For this review, take the finished solid that the model builds, in its own axes (mm). A direction names the side the tool comes from. Round coordinates to 2 decimals unless told otherwise and drop trailing zeros. Write each loop counter-clockwise with the first axis right and the second up, starting at its lowest first coordinate (ties: lowest second). Pieces come first, ordered by that corner, then holes. Notation, with made-up numbers: (15, -8.75) - (33, -8.75) arc R26 cw to (33, 11.25) - close; hole circle Ø2 at (9.25, 33.5). An arc over 180 degrees is marked (long way). One line per item, written item: value. Start each with the question number.
Q1. Tool access review of faces 1 (the face through (-24, -40, -7)), 2 (the face through (71.5, -0.6, -81.1)): name each direction out of +Z, -Z, +X, -X, +Y, -Y from which nothing blocks a thin tool from reaching the whole face with its end or side.
Q2. Add section A-A on x = 8. Write out the cut boundary in (y, z).
Q3. Add section D-D on z = -49. Write out the cut boundary in (x, y).
Q4. Add section C-C on x = -41.5. Write out the cut boundary in (y, z).
Q5. Add section B-B on y = -21. Write out the cut boundary in (x, z).
Q6. For probe 1 along Y at (x, z) = (-41.5, -0.7); probe 2 along Y at (x, z) = (9.5, -155), list the stretches that pass through material, from the lowest coordinate up.
Q7. Mouldability with a two-part tool opening along Y and no side actions: class faces 3 (the face through (-64.1, -10.9, -0.5)), 4 (the face through (62, -41, -7)), 5 (the face through (-1, -21, 0)) as +Y half, -Y half, draft (parallel to the pull), parting line (faces both ways), or undercut.
Q8. Clearance check with flat-ended pins moving along their axes: pin 1 Ø0.8 at (x, z) = (8.5, -0.5) entering from +Y (3 decimals); pin 2 Ø10 at (x, z) = (64, -4) entering from -Y; pin 3 Ø1.1 at (x, y) = (-24, -40.5) entering from -Z. State where each tip first meets the part, or that it passes through.
```python
from build123d import *

# Parameters (mm, degrees)
BASE_FLANGE1_START       = -71.5
BASE_FLANGE1_DEPTH       = 143
SKETCH6_W                = 39
SKETCH6_H                = 165
CUT_EXTRUDE1_DEPTH       = 1
SKETCH7_W                = 4
SKETCH7_H                = 46
CUT_EXTRUDE2_DEPTH       = 10
SKETCH8_R                = 2.6
CUT_EXTRUDE3_DEPTH       = 1
SKETCH9_W                = 16
SKETCH9_H                = 2
SKETCH9_W_2              = 8
SKETCH9_H_2              = 4.5
CUT_EXTRUDE4_DEPTH       = 185.66523766
SKETCH10_R               = 1.25
CUT_EXTRUDE5_DEPTH       = 1
EDGE_FLANGE1_START       = 56
EDGE_FLANGE1_DEPTH       = 13
EDGE_FLANGE1_2_DEPTH     = 0.5
EDGE_FLANGE1_START_2     = 68.5
EDGE_FLANGE1_3_DEPTH     = 0.5
EDGE_FLANGE1_START_3     = 56.5
EDGE_FLANGE1_4_OUTLINE_W = 1
EDGE_FLANGE1_4_OUTLINE_H = 9
EDGE_FLANGE1_4_DEPTH     = 12
EDGE_FLANGE2_START       = -30
EDGE_FLANGE2_DEPTH       = 13
EDGE_FLANGE2_2_DEPTH     = 0.5
EDGE_FLANGE2_START_2     = -17.5
EDGE_FLANGE2_3_DEPTH     = 0.5
EDGE_FLANGE2_START_3     = -29.5
EDGE_FLANGE2_4_OUTLINE_W = 1
EDGE_FLANGE2_4_OUTLINE_H = 9
EDGE_FLANGE2_4_DEPTH     = 12
SKETCH17_R               = 1.25
CUT_EXTRUDE6_DEPTH       = 1
FILLET1_R                = 2


# Read off the part's stored shape, not the designer's step: Base-Flange1, Edge-Flange1, Edge-Flange2
with BuildPart() as part:
    # Base-Flange1 outline → Base-Flange1 (new body)
    with BuildSketch(Plane(origin=(0, 0, 0), x_dir=(0, 0, -1), z_dir=(1, 0, 0)).offset(BASE_FLANGE1_START)):
        with BuildLine():
            Line((1, -1), (165, -1))
            Line((165, -1), (165, 0))
            Line((165, 0), (1, 0))
            ThreePointArc((1, 0), (0.292893219, -0.292893219), (0, -1))
            Line((0, -1), (0, -42))
            Line((0, -42), (1, -42))
            Line((1, -42), (1, -1))
        make_face()
    extrude(amount=BASE_FLANGE1_DEPTH)

    # Sketch6 → Cut-Extrude1 (cut)
    with BuildSketch(Plane(origin=(0, 0, 0), x_dir=(1, 0, 0), z_dir=(0, 1, 0))):
        with Locations((-52, 82.5)):
            Rectangle(SKETCH6_W, SKETCH6_H)
    extrude(amount=-CUT_EXTRUDE1_DEPTH, mode=Mode.SUBTRACT)

    # Sketch7 → Cut-Extrude2 (cut)
    with BuildSketch(Plane(origin=(0, 0, 0), x_dir=(1, 0, 0), z_dir=(0, 1, 0))):
        with Locations((-30.5, 142)):
            Rectangle(SKETCH7_W, SKETCH7_H)
    extrude(amount=-CUT_EXTRUDE2_DEPTH, mode=Mode.SUBTRACT)

    # Sketch8 → Cut-Extrude3 (cut)
    with BuildSketch(Plane.XY):
        with Locations((-61.5, -11)):
            Circle(SKETCH8_R)
        with Locations((-41.5, -31)):
            Circle(SKETCH8_R)
    extrude(amount=-CUT_EXTRUDE3_DEPTH, mode=Mode.SUBTRACT)

    # Sketch9 → Cut-Extrude4 (cut, through all)
    with BuildSketch(Plane.XY):
        with Locations((-6.5, -8)):
            Rectangle(SKETCH9_W, SKETCH9_H)
        with Locations((9.5, -8.75)):
            Rectangle(SKETCH9_W_2, SKETCH9_H_2)
    extrude(amount=-CUT_EXTRUDE4_DEPTH, mode=Mode.SUBTRACT)

    # Sketch10 → Cut-Extrude5 (cut)
    with BuildSketch(Plane(origin=(0, 0, 0), x_dir=(1, 0, 0), z_dir=(0, 1, 0))):
        with Locations(Location((66.5, 56, 0), (0, 0, 270))):
            Circle(SKETCH10_R)
        with Locations(Location((32.5, 135, 0), (0, 0, 270))):
            Circle(SKETCH10_R)
    extrude(amount=-CUT_EXTRUDE5_DEPTH, mode=Mode.SUBTRACT)

    # Edge-Flange1 outline → Edge-Flange1 (cut)
    with BuildSketch(Plane.YZ.offset(EDGE_FLANGE1_START)):
        with BuildLine():
            ThreePointArc((-41, -1), (-40.707106781, -0.292893219), (-40, 0))
            Line((-40, 0), (-42, 0))
            Line((-42, 0), (-42, -1))
            Line((-42, -1), (-41, -1))
        make_face()
    extrude(amount=EDGE_FLANGE1_DEPTH, mode=Mode.SUBTRACT)

    # Edge-Flange1 2 outline → Edge-Flange1 2 (cut)
    with BuildSketch(Plane.YZ.offset(EDGE_FLANGE1_START)):
        with BuildLine():
            Line((-39.5, -1), (-39.5, 0))
            Line((-39.5, 0), (-40, 0))
            ThreePointArc((-40, 0), (-40.707106781, -0.292893219), (-41, -1))
            Line((-41, -1), (-39.5, -1))
        make_face()
    extrude(amount=EDGE_FLANGE1_2_DEPTH, mode=Mode.SUBTRACT)

    # Edge-Flange1 3 outline → Edge-Flange1 3 (cut)
    with BuildSketch(Plane.YZ.offset(EDGE_FLANGE1_START_2)):
        with BuildLine():
            Line((-39.5, -1), (-39.5, 0))
            Line((-39.5, 0), (-40, 0))
            ThreePointArc((-40, 0), (-40.707106781, -0.292893219), (-41, -1))
            Line((-41, -1), (-39.5, -1))
        make_face()
    extrude(amount=EDGE_FLANGE1_3_DEPTH, mode=Mode.SUBTRACT)

    # Edge-Flange1 4 outline → Edge-Flange1 4 (add)
    with BuildSketch(Plane.YZ.offset(EDGE_FLANGE1_START_3)):
        with Locations((-40.5, -5.5)):
            Rectangle(EDGE_FLANGE1_4_OUTLINE_W, EDGE_FLANGE1_4_OUTLINE_H)
    extrude(amount=EDGE_FLANGE1_4_DEPTH)

    # Edge-Flange2 outline → Edge-Flange2 (cut)
    with BuildSketch(Plane.YZ.offset(EDGE_FLANGE2_START)):
        with BuildLine():
            ThreePointArc((-41, -1), (-40.707106781, -0.292893219), (-40, 0))
            Line((-40, 0), (-42, 0))
            Line((-42, 0), (-42, -1))
            Line((-42, -1), (-41, -1))
        make_face()
    extrude(amount=EDGE_FLANGE2_DEPTH, mode=Mode.SUBTRACT)

    # Edge-Flange2 2 outline → Edge-Flange2 2 (cut)
    with BuildSketch(Plane.YZ.offset(EDGE_FLANGE2_START)):
        with BuildLine():
            Line((-39.5, -1), (-39.5, 0))
            Line((-39.5, 0), (-40, 0))
            ThreePointArc((-40, 0), (-40.707106781, -0.292893219), (-41, -1))
            Line((-41, -1), (-39.5, -1))
        make_face()
    extrude(amount=EDGE_FLANGE2_2_DEPTH, mode=Mode.SUBTRACT)

    # Edge-Flange2 3 outline → Edge-Flange2 3 (cut)
    with BuildSketch(Plane.YZ.offset(EDGE_FLANGE2_START_2)):
        with BuildLine():
            Line((-39.5, -1), (-39.5, 0))
            Line((-39.5, 0), (-40, 0))
            ThreePointArc((-40, 0), (-40.707106781, -0.292893219), (-41, -1))
            Line((-41, -1), (-39.5, -1))
        make_face()
    extrude(amount=EDGE_FLANGE2_3_DEPTH, mode=Mode.SUBTRACT)

    # Edge-Flange2 4 outline → Edge-Flange2 4 (add)
    with BuildSketch(Plane.YZ.offset(EDGE_FLANGE2_START_3)):
        with Locations((-40.5, -5.5)):
            Rectangle(EDGE_FLANGE2_4_OUTLINE_W, EDGE_FLANGE2_4_OUTLINE_H)
    extrude(amount=EDGE_FLANGE2_4_DEPTH)

    # Sketch17 → Cut-Extrude6 (cut)
    with BuildSketch(Plane.XZ.offset(41)):
        with Locations(Location((-23.5, -5, 0), (0, 0, 270))):
            Circle(SKETCH17_R)
        with Locations(Location((62.5, -5, 0), (0, 0, 270))):
            Circle(SKETCH17_R)
    extrude(amount=-CUT_EXTRUDE6_DEPTH, mode=Mode.SUBTRACT)

    # Fillet1
    fillet1_edges = [part.edges().sort_by_distance(p)[0] for p in [
        (71.5, -42, -0.5),
        (71.5, -0.5, -165),
        (-28.5, -0.5, -165),
        (-28.5, -0.5, -119),
        (-32.5, -0.5, -119),
        (-71.5, -42, -0.5),
        (-71.5, -1, -0.5),
        (-29.5, -40.5, -10),
        (-17.5, -40.5, -10),
        (56.5, -40.5, -10),
        (68.5, -40.5, -10),
    ]]
    fillet(fillet1_edges, radius=FILLET1_R - 0.0001)  # a hair under: the kernel refuses the full size


solid = part.part
```
Result set:
1. face 1: -Z, +X, -X
1. face 2: +Z, -Z, +X, +Y, -Y
2. outline: (-42, -1) - (-11, -1) - (-11, 0) - (-42, 0) - close; (-6.5, -1) - (-1, -1) - (-1, -165) - (0, -165) - (0, -1) arc R1 ccw to (-1, 0) - (-6.5, 0) - close
3. outline: (-32.5, -1) - (71.5, -1) - (71.5, 0) - (-32.5, 0) - close
4. outline: (-42, -1) - (-33.6, -1) - (-33.6, 0) - (-42, 0) - close; (-28.4, -1) - (-1, -1) - (-1, 0) - (-28.4, 0) - close
5. outline: (-71.5, -1) - (71.5, -1) - (71.5, 0) - (-71.5, 0) - close
6. probe 1: y = -42 to -33.6, -28.4 to -1
6. probe 2: y = -1 to 0
7. face 3: undercut
7. face 4: -Y half
7. face 5: draft
8. pin 1: stops at y = -0.005
8. pin 2: stops at y = -41
8. pin 3: stops at z = -10
